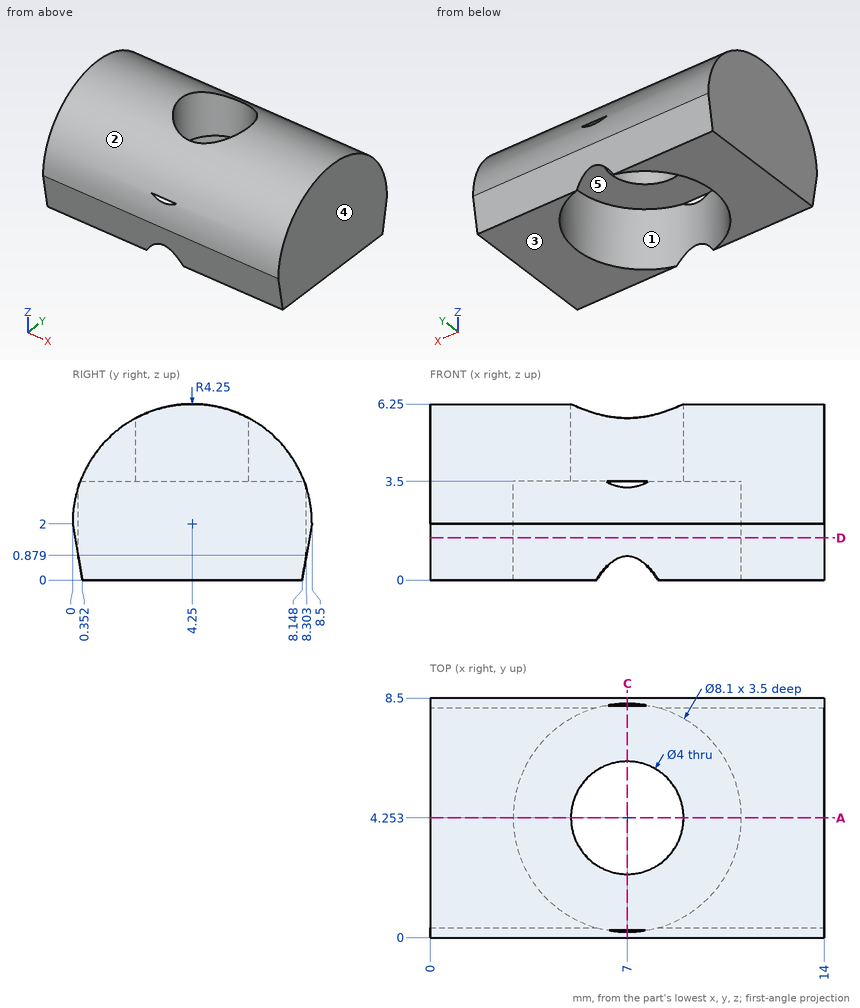
For this review, use the dimensioned drawing (mm, ordinates from the lowest corner) and the shaded views. A direction names the side the tool comes from. Coordinates: 2 decimals unless noted, no trailing zeros. Loops run counter-clockwise (first coordinate to the right, second up) from the corner with the lowest first, then second, coordinate; pieces in that order, holes last. Notation, with made-up numbers: (52.25, 20) -> (89.25, 20) arc R19 cw to (89.25, 33) -> close; hole circle Ø11 at (88.5, 25.25). An arc over 180 degrees is marked (long way). Use a Markdown table: item, result. Add a question column.
1. Draft analysis for pull direction X (two halves, no side actions). For the marked faces 3, 4 and 5, state which applies: pulls with the +X half, pulls with the -X half, needs draft (parallel to the pull), parting line crosses it, or undercut.
2. Clearance check with flat-ended pins moving along their axes: pin 1 Ø4.5 at (x, y) = (7, 4.25) entering from -Z; pin 2 Ø3 at (x, y) = (5, 7.5) entering from +Z. State where each tip first meets the part, or that it passes through.
3. To check wall thickness, follow line 1 (X direction, y = 3.5, z = 3); line 2 (Y direction, x = 9.5, z = 3.25) (1 decimal); line 3 (X direction, y = 3.75, z = 4.25) (1 decimal). State the ranges of each line that lie inside material, in increasing order.
4. Machinability: for the marked faces 1 and 2, which of the approach directions +Z, -Z, +X, -X, +Y, -Y give a long, thin tool a straight path to every point of the face, cutting with its end or side? Answer none if there is none.
5. Add section C-C on x = 7. Give the number of separate pieces and of enclosed holes in the cut face.
6. Add section A-A on y = 4.25. Write out the cut boundary in (x, z).
7. Add section D-D on z = 1.5. Write out the cut boundary in (x, y).
Returned:
| question | item | result |
|---|---|---|
| 1 | face 3 | needs draft |
| 1 | face 4 | pulls with the +X half |
| 1 | face 5 | undercut |
| 2 | pin 1 | stops at z = 3.5 |
| 2 | pin 2 | stops at z = 5.87 |
| 3 | line 1 | x = 0 to 3.02, 10.98 to 14 |
| 3 | line 2 | y = 0.2 to 1.1, 7.4 to 8.3 |
| 3 | line 3 | x = 0 to 5.1, 8.9 to 14 |
| 4 | face 1 | -Z |
| 4 | face 2 | +Z, +X, -X |
| 5 | separate pieces | 4 |
| 5 | enclosed holes | 0 |
| 6 | outline | (0, 0) -> (2.95, 0) -> (2.95, 3.5) -> (5, 3.5) -> (5, 6.25) -> (0, 6.25) -> close; (9, 3.5) -> (11.05, 3.5) -> (11.05, 0) -> (14, 0) -> (14, 6.25) -> (9, 6.25) -> close |
| 7 | outline | (0, 0.09) -> (14, 0.09) -> (14, 8.41) -> (0, 8.41) -> close; hole circle Ø8.1 at (7, 4.25) |
